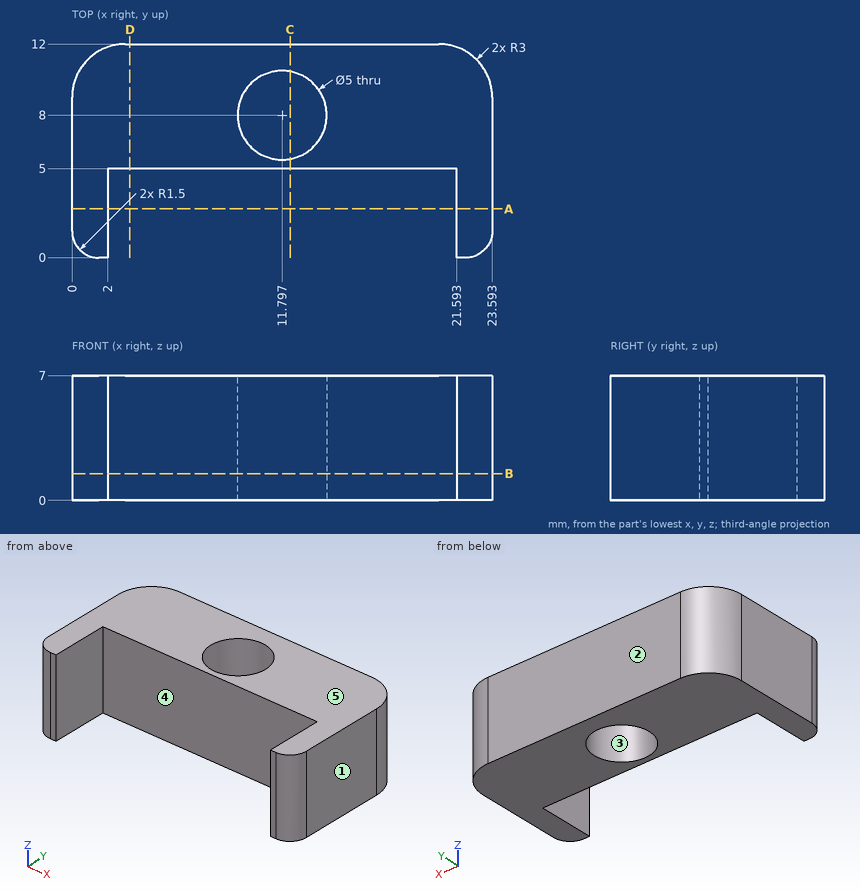
Input: dimensioned drawing with shaded views. Units: mm. Origin: part minimum x, y, z. A direction names the side the tool comes from. Round coordinates to 2 decimals unless told otherwise and drop trailing zeros. Loops run counter-clockwise (first coordinate to the right, second up) from the corner with the lowest first, then second, coordinate; pieces in that order, holes last. Notation, with made-up numbers: M 19,22.25 L 49,22.25 A23 ccw 49,50.25 Z; hole C 41,70.25 d1. An arc over 180 degrees is marked long. Answer in a Markdown table with one row per item. Add a question column.
1. Section B-B (z = 1.5). Output: boundary loops of the cut face in (x, y), and give its area (3 significant figures).
2. Section D-D (x = 3.25). Output: boundary loops of the cut face in (y, z).
3. Section C-C (x = 12.25). Output: boundary loops of the cut face in (y, z), and give its area (3 significant figures).
4. Section A-A (y = 2.75). Output: boundary loops of the cut face in (x, z), and give its area (3 significant figures).
5. Ray query, probe 1 along X at (y, z) = (2.5, 3.5); probe 2 along Y at (x, z) = (3.5, 4); probe 3 along X at (y, z) = (0.5, 6.25) (1 decimal). Return the intervals inside material, ascending.
6. Mould query, pull axis Y, two halves, no side actions, for the marked faces 1, 2 and 3. Classes: released by +Y, released by -Y, zero draft, split by the parting line, or undercut.
7. Contact query for a flat-ended pin moving along its axis: pin 1 (4 mm diameter, centred on x = 4.5, z = 5, fed in from -Y). Output: stop coordinate, or through.
8. Set-up query: the marked faces 4 and 5. Return all of +Z, -Z, +X, -X, +Y, -Y with unobstructed straight access to the full face (end or side cutting, diameter ignored); none if empty.
Values follow:
| question | item | result |
|---|---|---|
| 1 | outline | M 0,1.5 A1.5 ccw 1.5,0 L 2,0 L 2,5 L 21.59,5 L 21.59,0 L 22.09,0 A1.5 ccw 23.59,1.5 L 23.59,9 A3 ccw 20.59,12 L 3,12 A3 ccw 0,9 Z; hole C 11.8,8 d5 |
| 1 | area | 161 mm^2 |
| 2 | outline | M 5,0 L 12,0 L 12,7 L 5,7 Z |
| 3 | outline | M 5,0 L 5.54,0 L 5.54,7 L 5,7 Z; M 10.46,0 L 12,0 L 12,7 L 10.46,7 Z |
| 3 | area | 14.6 mm^2 |
| 4 | outline | M 0,0 L 2,0 L 2,7 L 0,7 Z; M 21.59,0 L 23.59,0 L 23.59,7 L 21.59,7 Z |
| 4 | area | 28.0 mm^2 |
| 5 | probe 1 | 0 to 2, 21.59 to 23.59 |
| 5 | probe 2 | 5 to 12 |
| 5 | probe 3 | 0.4 to 2, 21.6 to 23.2 |
| 6 | face 1 | zero draft |
| 6 | face 2 | released by +Y |
| 6 | face 3 | undercut |
| 7 | pin 1 | y = 5 |
| 8 | face 4 | +Z, -Z, -Y |
| 8 | face 5 | +Z, +X, -X, +Y, -Y |
